Geometry check sheet. Reference: the model listing, model coordinates, mm. A direction names the side the tool comes from. Round coordinates to 2 decimals unless told otherwise and drop trailing zeros. Write each loop counter-clockwise with the first axis right and the second up, starting at its lowest first coordinate (ties: lowest second). Pieces come first, ordered by that corner, then holes. Notation, with made-up numbers: (77, -32.5) - (84, -32.5) arc R36 cw to (84, 2.5) - close; hole circle Ø1 at (11, 62). An arc over 180 degrees is marked (long way). Return JSON: item names as keys, results as strings.
```python
from build123d import *

# Parameters (mm, degrees)
F0_W           = 56
F0_H           = 8
F1_DEPTH       = 120
F3_D           = 6
F5_D           = 6
F5_CBORE_D     = 11
F5_CBORE_DEPTH = 4


with BuildPart() as f1:
    # F0 (on Front) → F1 (new body)
    with BuildSketch(Plane.XZ):
        with Locations((28, 4)):
            Rectangle(F0_W, F0_H)
    extrude(amount=F1_DEPTH)

    # F3 (through all)
    with Locations(Plane.XY.offset(8)):
        with Locations((17, -14.5), (39, -14.5), (17, -105.5), (39, -105.5)):
            Hole(F3_D / 2)

    # F5 (through all)
    with Locations(Plane.XY.offset(8)):
        with Locations((8, -48), (8, -72), (48, -48), (48, -72)):
            CounterBoreHole(F5_D / 2, F5_CBORE_D / 2, F5_CBORE_DEPTH)


solid = f1.part
```
(1) Material ranges on line 1 along Y through (x, z) = (8, 6.9); line 2 along Y through (x, z) = (39, 2.25); line 3 along X through (y, z) = (-69.5, 6), recorded low to high. Write a range as [from, to].
Response values:
{"line 1": "y = [-120, -77.5], [-66.5, -53.5], [-42.5, 0]", "line 2": "y = [-120, -108.5], [-102.5, -17.5], [-11.5, 0]", "line 3": "x = [0, 3.1], [12.9, 43.1], [52.9, 56]"}
(2) Section check B-B, the plane y = -72. Enter the section's corners in (x, z).
Response values:
{"outline": "(0, 0) - (5, 0) - (5, 4) - (2.5, 4) - (2.5, 8) - (0, 8) - close; (11, 0) - (45, 0) - (45, 4) - (42.5, 4) - (42.5, 8) - (13.5, 8) - (13.5, 4) - (11, 4) - close; (51, 0) - (56, 0) - (56, 8) - (53.5, 8) - (53.5, 4) - (51, 4) - close"}
(3) Section check C-C, the plane z = 5.75. Give the number of separate pieces and of enclosed holes in the cut face, plus the area to 3 significant figures.
Response values:
{"separate pieces": "1", "enclosed holes": "8", "area": "6,230 mm^2"}
(4) Section check A-A, the plane x = 8. Enter the section's corners in (y, z), plus the area to 3 significant figures.
Response values:
{"outline": "(-120, 0) - (-75, 0) - (-75, 4) - (-77.5, 4) - (-77.5, 8) - (-120, 8) - close; (-69, 0) - (-51, 0) - (-51, 4) - (-53.5, 4) - (-53.5, 8) - (-66.5, 8) - (-66.5, 4) - (-69, 4) - close; (-45, 0) - (0, 0) - (0, 8) - (-42.5, 8) - (-42.5, 4) - (-45, 4) - close", "area": "824 mm^2"}
(5) Gauge pin test, flat ends, axial feed: pin 1 (5 mm diameter, centred on x = 17, y = -105.5, fed in from +Z); pin 2 (5.5 mm diameter, centred on x = 50, y = -47.5, fed in from +Z). Record the tip position at first contact, or that the pin passes through.
Response values:
{"pin 1": "passes through", "pin 2": "stops at z = 4"}
(6) Section check D-D, the plane y = -105.5. Enter the section's corners in (x, z).
Response values:
{"outline": "(0, 0) - (14, 0) - (14, 8) - (0, 8) - close; (20, 0) - (36, 0) - (36, 8) - (20, 8) - close; (42, 0) - (56, 0) - (56, 8) - (42, 8) - close"}
(7) Access from +Z, -Z, +X, -X, +Y, -Y to the whole of each face (thin tool, end or side, straight path). Record for faces 5 (the face through (10.4, -50.4, 4)), 6 (the face through (17.65, -108.43, 3.94)).
Response values:
{"face 5": "+Z", "face 6": "+Z, -Z"}
(8) Release check for a two-part mould opening along X. For faces 1 (the face through (0, -59, 4)), 2 (the face through (17.65, -17.43, 3.94)), 3 (the face through (28, -59, 8)), 4 (the face through (56, -59, 4)) record: pulls with the +X half, pulls with the -X half, needs draft (parallel to the pull), parting line crosses it, or undercut.
Response values:
{"face 1": "pulls with the -X half", "face 2": "undercut", "face 3": "needs draft", "face 4": "pulls with the +X half"}
